```python
from build123d import *

# Parameters (mm, degrees)
EXTRUDE_1_DEPTH     = 11
SKETCH_2_W          = 14
SKETCH_2_H          = 18
SKETCH_2_W_2        = 11
SKETCH_2_H_2        = 41
SKETCH_2_W_3        = 1.5
SKETCH_2_H_3        = 42
CUT_EXTRUDE_1_DEPTH = 28
FILLET_1_R          = 1
SKETCH_3_W          = 132.309001911
SKETCH_3_H          = 95.019202257
CUT_EXTRUDE_2_DEPTH = 76


with BuildPart() as part:
    # 草图1 → 凸台-拉伸1 (new, symmetric)
    with BuildSketch(Plane.XY):
        with BuildLine():
            Line((6, 50), (6, 0))
            ThreePointArc((6, 0), (0, -6), (-6, 0))
            Line((-6, 0), (-6, 50))
            ThreePointArc((-6, 50), (0, 56), (6, 50))
        make_face()
        with BuildLine():
            Line((2.2627417, 50), (1.13137085, 51.13137085))
            ThreePointArc((1.13137085, 51.13137085), (-1.6, 50), (1.13137085, 48.86862915))
            Line((1.13137085, 48.86862915), (2.2627417, 50))
        make_face(mode=Mode.SUBTRACT)
        with BuildLine():
            Line((2.2627417, 0), (1.13137085, 1.13137085))
            ThreePointArc((1.13137085, 1.13137085), (-1.6, 0), (1.13137085, -1.13137085))
            Line((1.13137085, -1.13137085), (2.2627417, 0))
        make_face(mode=Mode.SUBTRACT)
    extrude(amount=EXTRUDE_1_DEPTH, both=True)

    # 草图2 → 切除-拉伸1 (cut)
    with BuildSketch(Plane(origin=(6, 0, 0), x_dir=(0, 0, -1), z_dir=(1, 0, 0))):
        with Locations((0, 47)):
            Rectangle(SKETCH_2_W, SKETCH_2_H)
        with Locations((0, 14.5)):
            Rectangle(SKETCH_2_W_2, SKETCH_2_H_2)
        with Locations((-10.25, 15)):
            Rectangle(SKETCH_2_W_3, SKETCH_2_H_3)
        with Locations((10.25, 15)):
            Rectangle(SKETCH_2_W_3, SKETCH_2_H_3)
    extrude(amount=-CUT_EXTRUDE_1_DEPTH, mode=Mode.SUBTRACT)

    # 圆角1
    fillet_1_edges = [part.edges().sort_by_distance(p)[0] for p in [
        (0, 36, -11),
        (0, 38, -7),
        (0, 38, 7),
        (0, 36, 11),
    ]]
    fillet(fillet_1_edges, radius=FILLET_1_R)

    # 草图3 → 切除-拉伸2 (cut)
    with BuildSketch(Plane(origin=(0, 0, 5.5), x_dir=(-1, 0, 0), z_dir=(0, 0, -1))):
        with Locations((2.071719377, 26.254861983)):
            Rectangle(SKETCH_3_W, SKETCH_3_H)
    extrude(amount=CUT_EXTRUDE_2_DEPTH, mode=Mode.SUBTRACT)


solid = part.part
```
Verification items for the finished model (mm, model axes). A direction names the side the tool comes from. Coordinates: 2 decimals unless noted, no trailing zeros. Loops run counter-clockwise (first coordinate to the right, second up) from the corner with the lowest first, then second, coordinate; pieces in that order, holes last. Notation, with made-up numbers: (77.25, 17.5) - (131.25, 17.5) arc R10 cw to (131.25, 23.5) - close; hole circle Ø11 at (-35, 14). An arc over 180 degrees is marked (long way). Answer as a JSON object with one key per item and string values.
(1) Go/stop test with flat-tipped pins: pin 1 Ø3 at (x, z) = (4, 8.5) entering from +Y; pin 2 Ø1 at (x, z) = (3, 9.5) entering from -Y; pin 3 Ø2 at (x, z) = (-3, 7) entering from +Y. Record where each tip stops, or that it passes through.
Response:
{"pin 1": "stops at y = 55.45", "pin 2": "stops at y = -5.45", "pin 3": "stops at y = 55.66"}
(2) Scan lines: line 1 along Y through (x, z) = (0, 8.5); line 2 along Z through (x, y) = (4, 18.5); line 3 along Z through (x, y) = (-4.75, 44). Record each from-to range of solid material in increasing order.
Response:
{"line 1": "y = -6 to -1.6, 1.6 to 48.4, 51.6 to 56", "line 2": "z = 5.5 to 9.5", "line 3": "z = 7 to 11"}
(3) Mould release check, pull along X, two halves, no side actions. Record for faces 5 (the cylindrical face through (0, -6, 8)), 6 (the cylindrical face through (-0.084, 38.301, 6.715)), 7 (the flat face through (1.69, -0.57, 7.53)): pulls with the +X half, pulls with the -X half, needs draft (parallel to the pull), parting line crosses it, or undercut.
Response:
{"face 5": "parting line crosses it", "face 6": "needs draft", "face 7": "undercut"}
(4) Cross-section at D-D, the plane x = -2.5. Record the boundary of the cut face in (y, z).
Response:
{"outline": "(-5.45, 5.5) - (38, 5.5) - (38, 6) arc R1 cw to (39, 7) - (55.45, 7) - (55.45, 11) - (37, 11) arc R1 ccw to (36, 10) - (36, 9.5) - (-5.45, 9.5) - close"}
(5) Cross-section at A-A, the plane z = 8.65. Record the boundary of the cut face in (x, y), then the cut area to 3 significant figures.
Response:
{"outline": "(-6, 0) arc R6 ccw to (6, 0) - (6, 50) arc R6 ccw to (-6, 50) - close; hole (1.13, -1.13) - (2.26, 0) - (1.13, 1.13) arc R1.6 ccw (long way) to start; hole (1.13, 48.87) - (2.26, 50) - (1.13, 51.13) arc R1.6 ccw (long way) to start", "area": "696 mm²"}
(6) Cross-section at B-B, the plane x = 0. Record the boundary of the cut face in (y, z), then the cut area to 3 significant figures.
Response:
{"outline": "(-6, 5.5) - (-1.6, 5.5) - (-1.6, 9.5) - (-6, 9.5) - close; (1.6, 5.5) - (38, 5.5) - (38, 6) arc R1 cw to (39, 7) - (48.4, 7) - (48.4, 11) - (37, 11) arc R1 ccw to (36, 10) - (36, 9.5) - (1.6, 9.5) - close; (51.6, 7) - (56, 7) - (56, 11) - (51.6, 11) - close", "area": "225 mm²"}
(7) Access from +Z, -Z, +X, -X, +Y, -Y to the whole of each face (thin tool, end or side, straight path). Record for faces 1 (the cylindrical face through (0, 56, 9)), 2 (the flat face through (1.7, 50.56, 9.03)), 3 (the flat face through (0, 47, 7)), 4 (the flat face through (0, 15, 9.5)).
Response:
{"face 1": "+Z, -Z, +Y", "face 2": "+Z, -Z", "face 3": "-Z, +X, -X, +Y", "face 4": "+Z, +X, -X, -Y"}
(8) Cross-section at C-C, the plane y = 25.5. Record the boundary of the cut face in (x, z), then the cut area to 3 significant figures.
Response:
{"outline": "(-6, 5.5) - (6, 5.5) - (6, 9.5) - (-6, 9.5) - close", "area": "48.0 mm²"}
